Solid Edge part; units mm, degrees
sketch "Sketch1" plane through (0, 0, 0) normal (0, -1, 0) x (1, 0, 0)
  line L0 (-100, -30) -> (100, -30)
  line L1 (100, -30) -> (100, 30)
  line L2 (100, 30) -> (-100, 30)
  line L3 (-100, 30) -> (-100, -30)
  dimension "D1" = 100
  dimension "D2" = 100
extrude "Protrusion1" add sketch "Sketch1" against normal blind 2
sketch "Sketch2" plane through (0, 0, 0) normal (0, -1, 0) x (1, 0, 0)
  line L0 (-39.6222, 11.5432) -> (-48.7647, 28.7907)
  line L1 (-48.7647, 28.7907) -> (-68.9181, 28.7907)
  line L2 (-68.9181, 28.7907) -> (-78.6631, 12.1124)
  line L3 (-78.6631, 12.1124) -> (-65.8971, 12.1124)
  line L4 (-65.8971, 12.1124) -> (-62.8688, 18.0634)
  line L5 (-62.8688, 18.0634) -> (-55.6447, 18.0634)
  line L6 (-55.6447, 18.0634) -> (-51.8394, 12.1124)
  line L7 (-51.8394, 12.1124) -> (-55.6447, 5.4911)
  line L8 (-55.6447, 5.4911) -> (-62.8688, 5.4911)
  line L9 (-62.8688, 5.4911) -> (-62.8688, -5.6236)
  line L10 (-62.8688, -5.6236) -> (-55.2147, -5.6236)
  line L11 (-55.2147, -5.6236) -> (-51.8394, -11.6625)
  line L12 (-51.8394, -11.6625) -> (-55.2147, -18.0171)
  line L13 (-55.2147, -18.0171) -> (-62.8688, -18.0171)
  line L14 (-62.8688, -18.0171) -> (-65.8971, -11.6625)
  line L15 (-65.8971, -11.6625) -> (-78.6631, -11.6625)
  line L16 (-78.6631, -11.6625) -> (-68.9922, -28.7907)
  line L17 (-48.7647, -28.7907) -> (-68.9922, -28.7907)
  line L18 (-48.7647, -28.7907) -> (-39.6222, -12.3974)
  line L19 (-39.6222, -12.3974) -> (-45.6448, 0)
  line L20 (-45.6448, 0) -> (-39.6222, 11.5432)
  line L21 (-29.8239, 28.7907) -> (-39.0136, 11.3404)
  line L22 (-39.0136, 11.3404) -> (-27.2051, 11.3404)
  line L23 (-27.2051, 11.3404) -> (-23.5794, 17.7709)
  line L24 (-23.5794, 17.7709) -> (-16.2069, 17.7709)
  line L25 (-16.2069, 17.7709) -> (-12.7725, 11.3404)
  line L26 (-12.7725, 11.3404) -> (-16.2069, 5.3584)
  line L27 (-16.2069, 5.3584) -> (-23.5794, 5.3584)
  line L28 (-23.5794, 5.3584) -> (-23.5794, -5.3744)
  line L29 (-23.5794, -5.3744) -> (-16.2069, -5.3744)
  line L30 (-16.2069, -5.3744) -> (-12.7725, -11.9215)
  line L31 (-12.7725, -11.9215) -> (-16.2069, -18.0364)
  line L32 (-16.2069, -18.0364) -> (-23.5794, -18.0364)
  line L33 (-23.5794, -18.0364) -> (-27.2051, -11.9215)
  line L34 (-27.2051, -11.9215) -> (-39.0832, -11.9215)
  line L35 (-39.0832, -11.9215) -> (-39.0211, -12.3974)
  line L36 (-39.0211, -12.3974) -> (-29.8416, -28.7907)
  line L37 (-29.8416, -28.7907) -> (-9.9734, -28.7907)
  line L38 (-9.9734, -28.7907) -> (0, -11.7929)
  line L39 (0, -11.7929) -> (-6.8407, 0)
  line L40 (-6.8407, 0) -> (0, 11.8515)
  line L41 (0, 11.8515) -> (-9.9734, 28.7907)
  line L42 (-9.9734, 28.7907) -> (-29.8239, 28.7907)
  line L43 (9.4303, 28.7907) -> (0, 12.3815)
  line L44 (0, 12.3815) -> (0.2872, 11.8515)
  line L45 (0.2872, 11.8515) -> (12.5492, 11.8515)
  line L46 (12.5492, 11.8515) -> (15.7991, 18.0247)
  line L47 (15.7991, 18.0247) -> (23.265, 18.0247)
  line L48 (23.265, 18.0247) -> (26.8369, 11.8515)
  line L49 (26.8369, 11.8515) -> (23.265, 5.318)
  line L50 (23.265, 5.318) -> (15.7991, 5.318)
  line L51 (15.7991, 5.318) -> (15.7991, -5.632)
  line L52 (15.7991, -5.632) -> (23.265, -5.632)
  line L53 (23.265, -5.632) -> (26.7839, -11.7003)
  line L54 (26.7839, -11.7003) -> (23.265, -17.8487)
  line L55 (23.265, -17.8487) -> (15.768, -17.8487)
  line L56 (15.768, -17.8487) -> (12.2913, -11.7003)
  line L57 (0.3007, -11.6312) -> (12.2913, -11.7003)
  line L58 (0, -12.7084) -> (0.3007, -11.6312)
  line L59 (0, -12.7084) -> (9.391, -28.7907)
  line L60 (9.391, -28.7907) -> (29.5768, -28.7907)
  line L61 (29.5768, -28.7907) -> (39.4696, -11.7929)
  line L62 (39.4696, -11.7929) -> (32.5504, 0)
  line L63 (39.014, 12.1809) -> (32.5504, 0)
  line L64 (29.5768, 28.7907) -> (39.014, 12.1809)
  line L65 (29.5768, 28.7907) -> (9.4303, 28.7907)
  line L66 (39.3531, 11.3913) -> (49.0927, 28.7907)
  line L67 (68.964, 28.7907) -> (49.0927, 28.7907)
  line L68 (78.6631, 11.3946) -> (68.964, 28.7907)
  line L69 (55.3829, -28.7907) -> (78.6631, 11.3946)
  line L70 (42.8739, -28.7907) -> (55.3829, -28.7907)
  line L71 (56.0977, -5.4746) -> (42.8739, -28.7907)
  line L72 (49.0927, -5.4746) -> (56.0977, -5.4746)
  line L73 (49.0927, -5.4746) -> (39.3531, 11.3913)
  line L74 (51.7218, 11.7746) -> (55.3868, 5.6144)
  line L75 (55.3868, 5.6144) -> (62.6387, 5.6144)
  line L76 (62.6387, 5.6144) -> (66.3037, 11.7746)
  line L77 (66.3037, 11.7746) -> (62.6387, 17.9349)
  line L78 (62.6387, 17.9349) -> (55.3868, 17.9349)
  line L79 (55.3868, 17.9349) -> (51.7218, 11.7746)
extrude "ExtrudedProtrusion_3" add sketch "Sketch2" along normal blind 3
properties part number "BumbleB0912"
Work out the finished part from the listing and answer in its coordinate system (mm). A direction names the side the tool comes from. Give positions to 0.01 mm unless a question says otherwise; leave off trailing zeros. Order: outer loops, then holes, each group sorted by start corner. A loop starts at its lowest first (then second) coordinate and runs counter-clockwise, first axis right, second up. Notation, with made-up numbers: (-29, -33.75) -> (-13, -33.75) arc R10 ccw to (-13, -23.75) -> close; hole circle Ø2 at (-22.75, 14.25). An arc over 180 degrees is marked (long way). Answer as a JSON object with one key per item and string values. Group by question number.
1. Section B-B on x = -4.5 is taken. Determine the outline of the cut face in (y, z), plus the area to 3 significant figures.
2. Section C-C on z = 23 is taken. Determine the outline of the cut face in (x, y).
3. Section D-D on z = -23 is taken. Determine the outline of the cut face in (x, y).
4. Section A-A on y = -1.25 is taken. Count the separate pieces of the cut face and the enclosed holes in it, plus the area to 3 significant figures.
5. The mould has two halves that part along X. Classify faces 4 (the flat face through (4.63, -1.48, -20.64)), 5 (the flat face through (-19, -3, 0)): released by +X, released by -X, zero draft, split by the parting line, or undercut.
6. A tool of negligible diameter and unlimited length cuts with its end or side. For faces 1 (the flat face through (-44.13, -1.48, 20.05)), 2 (the flat face through (34.454, -1.479, -20.411)), 3 (the flat face through (59, 0, 12)), from which of +Z, -Z, +X, -X, +Y, -Y can it reach the whole face along a straight path? Write none if from no direction.
7. Flat-ended cylindrical pins translate along their axes: pin 1 Ø1.5 at (x, y) = (-58.5, -1) entering from +Z; pin 2 Ø1.5 at (x, y) = (-19.5, -1) entering from -Z; pin 3 Ø0.9 at (x, y) = (8.5, -1.5) entering from -Z. Find the tip coordinate at first contact, or state that the pin passes through.
8. Consider line 1 along X through (y, z) = (-1.6, -6); line 2 along X through (y, z) = (-0.2, -27); line 3 along X through (y, z) = (-1, 9). Determine where each line is inside the solid, lowest interval first. Write a range as [from, to].
Result sheet:
{
 "1": {"outline": "(-3, -19.46) -> (0, -19.46) -> (0, -30) -> (2, -30) -> (2, 30) -> (0, 30) -> (0, 19.49) -> (-3, 19.49) -> (-3, 4.06) -> (0, 4.06) -> (0, -4.04) -> (-3, -4.04) -> close", "area": "213 mm^2"},
 "2": {"outline": "(-100, 0) -> (-72.3, 0) -> (-72.3, -3) -> (-45.7, -3) -> (-45.7, 0) -> (-32.87, 0) -> (-32.87, -3) -> (-6.56, -3) -> (-6.56, 0) -> (6.1, 0) -> (6.1, -3) -> (32.87, -3) -> (32.87, 0) -> (45.85, 0) -> (45.85, -3) -> (72.19, -3) -> (72.19, 0) -> (100, 0) -> (100, 2) -> (-100, 2) -> close"},
 "3": {"outline": "(-100, 0) -> (-72.26, 0) -> (-72.26, -3) -> (-45.54, -3) -> (-45.54, 0) -> (-33.08, 0) -> (-33.08, -3) -> (-6.58, -3) -> (-6.58, 0) -> (6.01, 0) -> (6.01, -3) -> (32.95, -3) -> (32.95, 0) -> (46.16, 0) -> (46.16, -3) -> (58.74, -3) -> (58.74, 0) -> (100, 0) -> (100, 2) -> (-100, 2) -> close"},
 "4": {"separate pieces": "4", "enclosed holes": "1", "area": "4,880 mm^2"},
 "5": {"face 4": "undercut", "face 5": "zero draft"},
 "6": {"face 1": "+Z, -Y", "face 2": "-Z, -Y", "face 3": "-Y"},
 "7": {"pin 1": "stops at z = 28.79", "pin 2": "stops at z = -28.79", "pin 3": "stops at z = -28.04"},
 "8": {"line 1": "x = [-55, -42.73], [-15.88, -3.36], [23.48, 36.07], [55.8, 68.59]", "line 2": "x = [-70, -47.77], [-30.84, -8.92], [8.35, 30.62], [43.89, 56.42]", "line 3": "x = [-53.63, -40.95], [-14.12, -1.65], [25.28, 37.33], [40.73, 53.37], [64.65, 77.28]"}
}
